Source: CAD feature listing. Evaluate the final solid. Frame: model axes, mm. A direction names the side the tool comes from. Give positions to 0.01 mm unless a question says otherwise; leave off trailing zeros. Order: outer loops, then holes, each group sorted by start corner. A loop starts at its lowest first (then second) coordinate and runs counter-clockwise, first axis right, second up.
1) Section B-B, the plane x = -3. Return loops of the section in (y, z).
2) First-contact query: P1, Ø2, axis at x = -0.5, y = 4, coming from the +Z side; P2, Ø1, axis at y = 25.5, z = -3, coming from the -X side; P3, Ø6.5, axis at x = -3.5, z = 3, coming from the -Y side; P4, Ø5.5, axis at y = -8, z = 1, coming from the +X side. Flat tips, straight axial feed; report the tip coordinate or a pass-through.
3) Material intervals for line 1 (X direction, y = 27.5, z = -11.5); line 2 (Y direction, x = 4, z = -0.75); line 3 (Z direction, x = 0.5, y = 1.5), sorted ascending.
4) Section C-C, the plane y = 20. Return loops of the section in (x, z).
5) Section A-A, the plane z = 0.75. Return loops of the section in (x, y), plus the area to 3 significant figures.
6) Access query for faces 4 (the face through (0, 3, -4.899)), 5 (the face through (0, -7, -5)), 6 (the face through (0, -7, 5)), 7 (the face through (-1, 18, 0)). Directions: +Z, -Z, +X, -X, +Y, -Y. A direction counts if a zero-diameter tool reaches every point of the face in a straight line with its end or side. Return the directions, or none.
7) Draft query along Y for faces 1 (the face through (0, 3, 4.899)), 2 (the face through (1, 18, 0)), 3 (the face through (-3, -1, 1)). Return one class per face: released by +Y, released by -Y, zero draft, split by the parting line, or undercut.
```python
from build123d import *

# Parameters (mm, degrees)
BOSS_EXTRUDE1_DEPTH = 13
SKETCH1_3_R         = 5
SKETCH1_3_R_2       = 2
BOSS_EXTRUDE2_DEPTH = 1
SKETCH1_5_W         = 2
SKETCH1_5_H         = 9.797958972
BOSS_EXTRUDE3_DEPTH = 20
SKETCH2_R           = 15
BOSS_EXTRUDE4_DEPTH = 2


with BuildPart() as part:
    # Sketch1 → Boss-Extrude1 (new body)
    with BuildSketch(Plane(origin=(0, 0, 0), x_dir=(1, 0, 0), z_dir=(0, 1, 0))):
        with BuildLine():
            Line((2.5, 2.5), (2.5, -2.5))
            ThreePointArc((2.5, -2.5), (0, -5), (-2.5, -2.5))
            Line((-2.5, -2.5), (-2.5, 2.5))
            ThreePointArc((-2.5, 2.5), (0, 5), (2.5, 2.5))
        make_face()
    extrude(amount=-BOSS_EXTRUDE1_DEPTH)

    # Sketch1_3 → Boss-Extrude2 (add)
    with BuildSketch(Plane(origin=(0, 0, 0), x_dir=(1, 0, 0), z_dir=(0, 1, 0))):
        Circle(SKETCH1_3_R)
        with Locations((0.435778714, -4.98097349)):
            Circle(SKETCH1_3_R_2)
        with Locations((-4.98097349, 0.435778714)):
            Circle(SKETCH1_3_R_2)
        with Locations((3.535533906, 3.535533906)):
            Circle(SKETCH1_3_R_2)
    extrude(amount=-BOSS_EXTRUDE2_DEPTH)

    # Sketch1_5 → Boss-Extrude3 (add)
    with BuildSketch(Plane(origin=(0, 0, 0), x_dir=(1, 0, 0), z_dir=(0, 1, 0))):
        Rectangle(SKETCH1_5_W, SKETCH1_5_H)
    extrude(amount=BOSS_EXTRUDE3_DEPTH)

    # Sketch2 → Boss-Extrude4 (add)
    with BuildSketch(Plane.ZY.offset(1)):
        with Locations((0, 20)):
            Circle(SKETCH2_R)
    extrude(amount=-BOSS_EXTRUDE4_DEPTH)


solid = part.part
```
From the geometry:
1. outline: (-1, -4) - (0, -4) - (0, 4) - (-1, 4) - close
2. P1: stops at z = 4.9
2. P2: stops at x = -1
2. P3: stops at y = -13
2. P4: stops at x = 2.5
3. line 1: x = -1 to 1
3. line 2: y = -1 to 0
3. line 3: z = -4.9 to 4.9
4. outline: (-1, -15) - (1, -15) - (1, 15) - (-1, 15) - close
5. outline: (-6.59, -1) - (-2.5, -1) - (-2.5, -13) - (2.5, -13) - (2.5, -1) - (4.94, -1) - (4.94, 0) - (1, 0) - (1, 34.98) - (-1, 34.98) - (-1, 0) - (-6.59, 0) - close
5. area: 141 mm2
6. face 4: -Z, +X, -X
6. face 5: -Z, -Y
6. face 6: +Z, -Y
6. face 7: +Z, -Z, -X, +Y
7. face 1: undercut
7. face 2: zero draft
7. face 3: released by -Y
